Job drawing, mm, ordinate dimensions from the low corner. One solid piece. A direction names the side the tool comes from. Coordinates: 2 decimals unless noted, no trailing zeros. Write each loop counter-clockwise with the first axis right and the second up, starting at its lowest first coordinate (ties: lowest second). Pieces come first, ordered by that corner, then holes. Notation, with made-up numbers: (76.5, -4.5) - (133.5, -4.5) arc R25 ccw to (133.5, 27.5) - close; hole circle Ø11 at (51, -34.5). An arc over 180 degrees is marked (long way). Use a Markdown table: item, result.
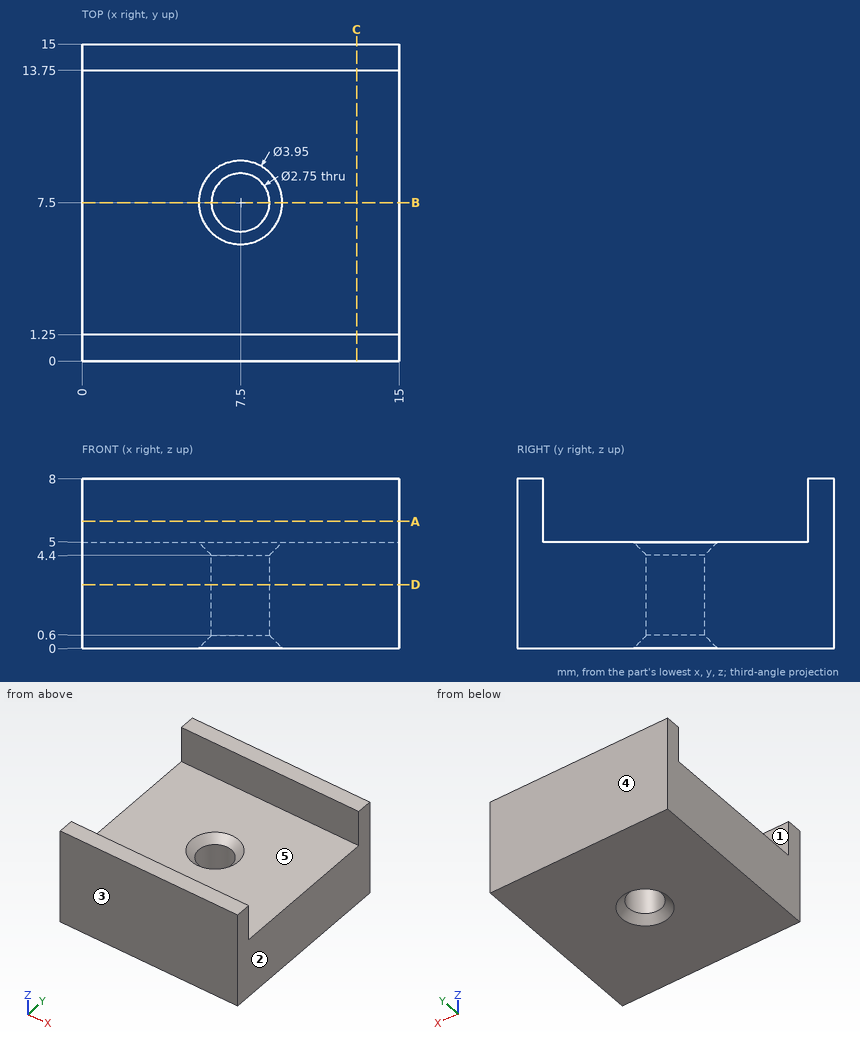
Item 1: Which spindle directions (+Z, -Z, +X, -X, +Y, -Y) get a long thin tool onto all of the face, cutting with end or side? Do the marked faces 4 and 5. Say none if no direction does.
From the geometry:
| item | result |
|---|---|
| face 4 | +Z, -Z, +X, -X, +Y |
| face 5 | +Z, +X, -X |
Item 2: Band-saw the part on C-C, the plane x = 13. Give the cut face in (y, z).
From the geometry:
| item | result |
|---|---|
| outline | (0, 0) - (15, 0) - (15, 8) - (13.75, 8) - (13.75, 5) - (1.25, 5) - (1.25, 8) - (0, 8) - close |
Item 3: Drop a flat-ended pin along its axis: P1, Ø4, axis at x = 7.5, y = 5, coming from the +Z side. Give the stop position or say it passes through.
From the geometry:
| item | result |
|---|---|
| P1 | z = 5 |
Item 4: Drill centre lines: probe 1 along Y at (x, z) = (7.5, 2.2) (3 decimals); probe 2 along Y at (x, z) = (1.75, 6.5). Where is each one in solid material? Low to high.
From the geometry:
| item | result |
|---|---|
| probe 1 | 0 to 6.125, 8.875 to 15 |
| probe 2 | 0 to 1.25, 13.75 to 15 |
Item 5: Band-saw the part on A-A, the plane z = 6. Give the cut face in (x, y).
From the geometry:
| item | result |
|---|---|
| outline | (0, 0) - (15, 0) - (15, 1.25) - (0, 1.25) - close; (0, 13.75) - (15, 13.75) - (15, 15) - (0, 15) - close |
Item 6: Two-plate mould, pull along Y, no slides. Class the marked faces 1, 2 and 3: pulls with the +Y half, pulls with the -Y half, needs draft (parallel to the pull), parting line crosses it, or undercut.
From the geometry:
| item | result |
|---|---|
| face 1 | undercut |
| face 2 | needs draft |
| face 3 | pulls with the -Y half |
Item 7: Band-saw the part on D-D, the plane z = 3. Give the cut face in (x, y) (3 decimals).
From the geometry:
| item | result |
|---|---|
| outline | (0, 0) - (15, 0) - (15, 15) - (0, 15) - close; hole circle Ø2.75 at (7.5, 7.5) |
Item 8: Band-saw the part on B-B, the plane y = 7.5. Give the cut face in (x, z) (3 decimals), then the cut area to 3 significant figures.
From the geometry:
| item | result |
|---|---|
| outline | (0, 0) - (5.525, 0) - (6.125, 0.6) - (6.125, 4.4) - (5.525, 5) - (0, 5) - close; (8.875, 0.6) - (9.475, 0) - (15, 0) - (15, 5) - (9.475, 5) - (8.875, 4.4) - close |
| area | 60.5 mm^2 |
